The drawing under review shows one solid part. Ordinate dimensions are in mm from its lowest x, y, z. A direction names the side the tool comes from. Coordinates: 2 decimals unless noted, no trailing zeros. Write each loop counter-clockwise with the first axis right and the second up, starting at its lowest first coordinate (ties: lowest second). Pieces come first, ordered by that corner, then holes.
Q1. Take a section at C-C (y = 8). Give the boundary of the cut face in (x, z), and give its area (3 significant figures).
Q2. Insertion check: pin 1 (1.5 mm diameter, centred on x = 20, y = 13.5, fed in from +Z); pin 2 (2 mm diameter, centred on x = 4, y = 9, fed in from -Z); pin 3 (1 mm diameter, centred on x = 13, z = 3.5, fed in from +Y); pin 4 (2 mm diameter, centred on x = 12, y = 14.5, fed in from -Z). Each pin has a flat end and moves straight along its axis. Give the tip position at first contact, or say it passes through.
Q3. Take a section at A-A (x = 12.5). Give the boundary of the cut face in (y, z).
Q4. Take a section at D-D (z = 2). Give the boundary of the cut face in (x, y) (1 decimal), and give its area (3 significant figures).
Q5. For probe 1 along Y at (x, z) = (3, 26); probe 2 along X at (y, z) = (14.25, 20); probe 3 along Z at (x, y) = (7.5, 15.5), list the stretches that pass through material, from the lowest coordinate up.
Q6. Take a section at B-B (z = 19.5). Give the boundary of the cut face in (x, y) (1 decimal), and give its area (3 significant figures).
Q7. Machinability: for the marked faces 1, 2, 3 and 4, which of the approach directions +Z, -Z, +X, -X, +Y, -Y give a long, thin tool a straight path to every point of the face, cutting with its end or side? Answer none if there is none.
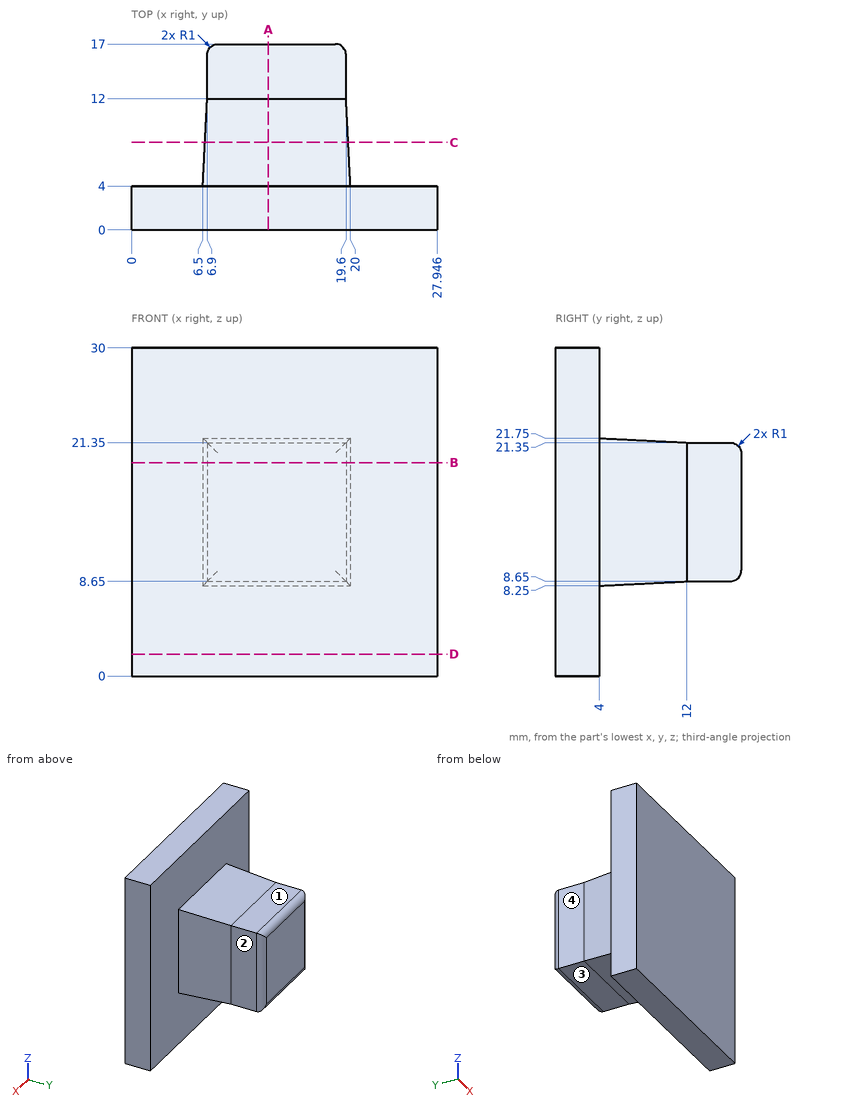
Response:
1. outline: (6.7, 8.45) - (19.8, 8.45) - (19.8, 21.55) - (6.7, 21.55) - close
1. area: 172 mm2
2. pin 1: stops at z = 21.35
2. pin 2: passes through
2. pin 3: stops at y = 4
2. pin 4: stops at z = 8.65
3. outline: (0, 0) - (4, 0) - (4, 8.25) - (12, 8.65) - (16, 8.65) arc R1 ccw to (17, 9.65) - (17, 20.35) arc R1 ccw to (16, 21.35) - (12, 21.35) - (4, 21.75) - (4, 30) - (0, 30) - close
4. outline: (0, 0) - (27.9, 0) - (27.9, 4) - (0, 4) - close
4. area: 112 mm2
5. probe 1: y = 0 to 4
5. probe 2: x = 6.9 to 19.6
5. probe 3: z = 8.65 to 21.35
6. outline: (0, 0) - (27.9, 0) - (27.9, 4) - (20, 4) - (19.6, 12) - (19.6, 16) arc R1 ccw to (18.6, 17) - (7.9, 17) arc R1 ccw to (6.9, 16) - (6.9, 12) - (6.5, 4) - (0, 4) - close
6. area: 280 mm2
7. face 1: +Z, +X, -X, +Y
7. face 2: +Z, -Z, +X, +Y
7. face 3: -Z, +X, -X, +Y
7. face 4: +Z, -Z, -X, +Y
